from build123d import *

# Parameters (mm, degrees)
BOSS_EXTRUDE1_DEPTH   = 12.2
SKETCH1_W             = 2
SKETCH1_H             = 22.4
BOSS_EXTRUDE1_2_DEPTH = 12.2
SKETCH1_4_W           = 1
SKETCH1_4_H           = 22.4
BOSS_EXTRUDE2_DEPTH   = 2


with BuildPart() as part:
    # Sketch1 → Boss-Extrude1 (new body)
    with BuildSketch(Plane(origin=(0, 0, 0), x_dir=(1, 0, 0), z_dir=(0, 1, 0))):
        Polygon((0, 5), (0, 0), (6, 0), (6, -11.5), (0.8, -11.5), (0.8, -13.4), (4.5, -13.4), (4.5, -17.4), (8.5, -17.4), (8.5, 5), align=None)
    extrude(amount=BOSS_EXTRUDE1_DEPTH)



with BuildPart() as body_2:
    # Sketch1 → Boss-Extrude1 2 (new body)
    with BuildSketch(Plane(origin=(0, 0, 0), x_dir=(1, 0, 0), z_dir=(0, 1, 0))):
        with Locations((10.5, -6.2)):
            Rectangle(SKETCH1_W, SKETCH1_H)
    extrude(amount=BOSS_EXTRUDE1_2_DEPTH)


with BuildPart() as part_1:
    add(part.part)

    add(body_2.part)  # Boss-Extrude2 merges body 2
    # Sketch1<4> → Boss-Extrude2 (add)
    with BuildSketch(Plane(origin=(0, 0, 0), x_dir=(1, 0, 0), z_dir=(0, 1, 0))):
        with Locations((9, -6.2)):
            Rectangle(SKETCH1_4_W, SKETCH1_4_H)
    extrude(amount=BOSS_EXTRUDE2_DEPTH)


solid = part_1.part
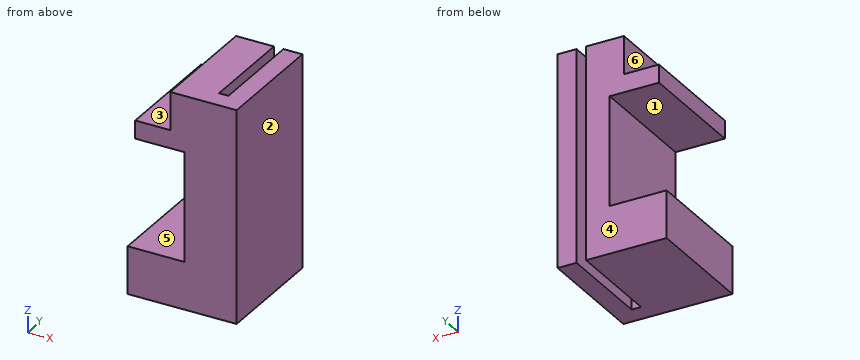
Geometry: final body of the model. Coordinates: model frame, mm. Face numbers are marked on the shaded views. A direction names the side the tool comes from. Round coordinates to 2 decimals unless told otherwise and drop trailing zeros. Loops run counter-clockwise (first coordinate to the right, second up) from the corner with the lowest first, then second, coordinate; pieces in that order, holes last.
Q1. Pull-direction query (Z, two-part tool) for the marked faces 1, 2 and 3; classes: released by +Z, released by -Z, zero draft, split by the parting line, or undercut.
Q2. Pin query (flat end, axial travel): P1, Ø1, axis at y = 3, z = 7, coming from the -X side; P2, Ø5, axis at y = 7.5, z = 11.5, coming from the -X side; P3, Ø0.5, axis at x = 9, z = 5, coming from the +Y side. Return the tip coordinate at first contact, or that it passes through.
Q3. Section B-B on y = 10.75. Return loops of the section in (x, z).
Q4. Section D-D on y = 1. Return loops of the section in (x, z), plus the area to 3 significant figures.
Q5. Section C-C on z = 9.25. Return loops of the section in (x, y), plus the area to 3 significant figures.
Q6. Section A-A on x = 5.25. Return loops of the section in (y, z), plus the area to 3 significant figures.
Q7. Material intervals for L1, parallel to X at y = 5.75, z = -3.5; L2, parallel to Z at x = 1, y = 5.25; L3, parallel to X at y = 10, z = 13.25, sorted ascending.
Q8. Access query for the marked faces 4, 5 and 6. Directions: +Z, -Z, +X, -X, +Y, -Y. A direction counts if a zero-diameter tool reaches every point of the face in a straight line with its end or side. Return the directions, or none.
Evaluation:
1. face 1: undercut
1. face 2: zero draft
1. face 3: released by +Z
2. P1: stops at x = 6
2. P2: stops at x = 0.8
2. P3: stops at y = 2
3. outline: (0, -5) - (8.5, -5) - (8.5, 17.4) - (4.5, 17.4) - (4.5, 13.4) - (0.8, 13.4) - (0.8, 11.5) - (6, 11.5) - (6, 0) - (0, 0) - close; (9.5, -5) - (11.5, -5) - (11.5, 17.4) - (9.5, 17.4) - close
4. outline: (0, -5) - (11.5, -5) - (11.5, 17.4) - (4.5, 17.4) - (4.5, 13.4) - (0.8, 13.4) - (0.8, 11.5) - (6, 11.5) - (6, 0) - (0, 0) - close
4. area: 169 mm2
5. outline: (6, 0) - (11.5, 0) - (11.5, 12.2) - (9.5, 12.2) - (9.5, 2) - (8.5, 2) - (8.5, 12.2) - (6, 12.2) - close
5. area: 56.9 mm2
6. outline: (0, -5) - (12.2, -5) - (12.2, 0) - (0, 0) - close; (0, 11.5) - (12.2, 11.5) - (12.2, 17.4) - (0, 17.4) - close
6. area: 133 mm2
7. L1: x = 0 to 8.5, 9.5 to 11.5
7. L2: z = -5 to 0, 11.5 to 13.4
7. L3: x = 0.8 to 8.5, 9.5 to 11.5
8. face 4: +Z, -Z, +X, -X, +Y
8. face 5: -X, +Y, -Y
8. face 6: +Z, -X, +Y, -Y
